The model under review builds one solid part; all positions refer to its coordinate system, in mm. A direction names the side the tool comes from. Round coordinates to 2 decimals unless told otherwise and drop trailing zeros. Write each loop counter-clockwise with the first axis right and the second up, starting at its lowest first coordinate (ties: lowest second). Pieces come first, ordered by that corner, then holes. Notation, with made-up numbers: M 74.5,41.25 L 115.5,41.25 A18 cw 115.5,57.25 Z; hole C -0.75,58.5 d9. An arc over 180 degrees is marked long. Write item = value, one per line. Start each with the question number.
Item 1: Take a section at B-B, the plane y = 7.25. Give the boundary of the cut face in (x, z).
Item 2: The part is to be moulded in two halves that separate along X. For faces 6 (the flat face through (-15, 10, 3)), 7 (the flat face through (-7, 6, 3)), 8 (the flat face through (-11.5, 6, 3)), say which applies: +X half, -X half, draft (parallel to the pull), parting line (faces both ways), or undercut.
Item 3: To check wall thickness, follow line 1 along X through (y, z) = (0.6, 3); line 2 along X through (y, z) = (3.25, 2); line 3 along Y through (x, z) = (-16, 3.25). State the ranges of each line that lie inside material, in increasing order.
Item 4: Take a section at C-C, the plane y = -7.5. Give the boundary of the cut face in (x, z).
Item 5: Take a section at A-A, the plane x = -21.5. Give the boundary of the cut face in (y, z).
Item 6: Take a section at D-D, the plane z = 3.75. Give the number of separate pieces and of enclosed holes in the cut face, plus the area to 3 significant figures.
Item 7: Tool access review of faces 1 (the flat face through (-17.5, 6, 3)), 2 (the flat face through (-24.5, 1, 3)), 3 (the flat face through (-10, 10, 3)), 4 (the flat face through (-5, 3, 3)), 5 (the flat face through (-12, 3, 3)): name each direction out of +Z, -Z, +X, -X, +Y, -Y from which nothing blocks a thin tool from reaching the whole face with its end or side.
Item 8: For pin 1 Ø1.8 at (y, z) = (7.5, 2) entering from -X; pin 2 Ø1.8 at (x, z) = (-14.5, 4.5) entering from -Y; pin 3 Ø1 at (x, z) = (-17.5, 5) entering from -Y; pin 4 Ø1.5 at (y, z) = (-4.5, 4.5) entering from +X, all flat-tipped, find the tip position at first contact; note any pin that passes through.
from build123d import *

# Parameters (mm, degrees)
CROQUIS1_W              = 24.5
CROQUIS1_H              = 6
CROQUIS1_R              = 1.75
SALIENTE_EXTRUIR1_DEPTH = 3
CROQUIS2_W              = 4.5
CROQUIS2_H              = 6
SALIENTE_EXTRUIR2_DEPTH = 7
REDONDEO1_SIZE          = 1
CROQUIS3_R              = 0.05
SALIENTE_EXTRUIR3_DEPTH = 11


with BuildPart() as part:
    # Croquis1 → Saliente-Extruir1 (new body)
    with BuildSketch(Plane(origin=(0, 0, 0), x_dir=(1, 0, 0), z_dir=(0, 1, 0))):
        with Locations((-12.25, -3)):
            Rectangle(CROQUIS1_W, CROQUIS1_H)
        with Locations(Location((-21.5, -3, 0), (0, 0, 270))):
            Circle(CROQUIS1_R, mode=Mode.SUBTRACT)
        with Locations(Location((-3, -3, 0), (0, 0, 90))):
            Circle(CROQUIS1_R, mode=Mode.SUBTRACT)
    extrude(amount=SALIENTE_EXTRUIR1_DEPTH)

    # Croquis2 → Saliente-Extruir2 (add)
    with BuildSketch(Plane(origin=(0, 3, 0), x_dir=(1, 0, 0), z_dir=(0, 1, 0))):
        with Locations((-15.25, -3)):
            Rectangle(CROQUIS2_W, CROQUIS2_H)
        with Locations((-9.25, -3)):
            Rectangle(CROQUIS2_W, CROQUIS2_H)
    extrude(amount=SALIENTE_EXTRUIR2_DEPTH)

    # Redondeo1
    # a fillet whose section is not a circle: 1 mm, written as the material it takes off along each edge
    with BuildSketch(Plane(origin=(-7, 10, -2.5), x_dir=(0, -1, 0), z_dir=(0, 0, 1))) as redondeo1_piece_1:
        with BuildLine():
            Bezier((REDONDEO1_SIZE, 0), (0, 0), (0, -REDONDEO1_SIZE), weights=[1, 0.707106781, 1])
            Line((0, -REDONDEO1_SIZE), (0, 0))
            Line((0, 0), (REDONDEO1_SIZE, 0))
        make_face()
    extrude(amount=11, mode=Mode.SUBTRACT)

    # Croquis3 → Saliente-Extruir3 (add)
    with BuildSketch(Plane.XZ):
        with Locations(Location((-15.25, 4.5, 0), (0, 0, 270))):
            Circle(CROQUIS3_R)
        with Locations(Location((-15.25, 1.5, 0), (0, 0, 90))):
            Circle(CROQUIS3_R)
        with Locations(Location((-9.25, 4.5, 0), (0, 0, 90))):
            Circle(CROQUIS3_R)
        with Locations(Location((-9.25, 1.5, 0), (0, 0, 270))):
            Circle(CROQUIS3_R)
    extrude(amount=SALIENTE_EXTRUIR3_DEPTH)


solid = part.part
Response values:
q1.outline = M -17.5,0 L -13,0 L -13,6 L -17.5,6 Z; M -11.5,0 L -7,0 L -7,6 L -11.5,6 Z
q2.face_6 = draft
q2.face_7 = +X half
q2.face_8 = undercut
q3.line_1 = -24.5 to -23.25, -19.75 to -4.75, -1.25 to 0
q3.line_2 = -17.5 to -13, -11.5 to -7
q3.line_3 = 0 to 10
q4.outline = C -15.25,1.5 d0.1; C -15.25,4.5 d0.1; C -9.25,1.5 d0.1; C -9.25,4.5 d0.1
q5.outline = M 0,0 L 3,0 L 3,1.25 L 0,1.25 Z; M 0,4.75 L 3,4.75 L 3,6 L 0,6 Z
q6.separate_pieces = 3
q6.enclosed_holes = 0
q6.area = 117 mm2
q7.face_1 = +Z, -Z, -X, +Y
q7.face_2 = +Z, -Z, -X, +Y, -Y
q7.face_3 = +Z, -Z, +X, -X, +Y
q7.face_4 = +Z, -Z, +X, +Y
q7.face_5 = +Z, -Z, +Y
q8.pin_1 = -17.5
q8.pin_2 = -11
q8.pin_3 = 0
q8.pin_4 = -9.2
